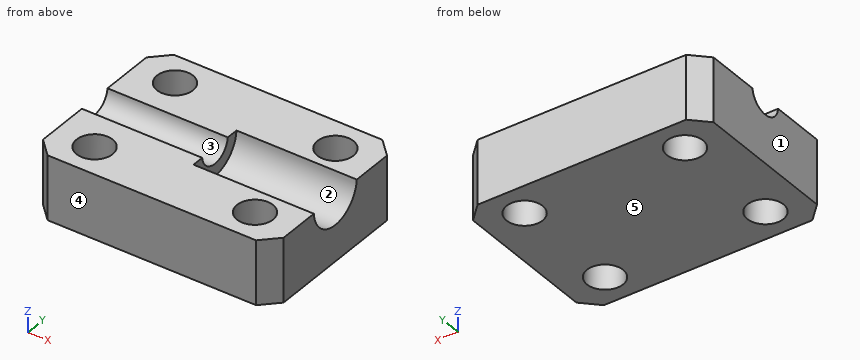
```python
from build123d import *

# Parameters (mm, degrees)
SKETCH2_R           = 2.25
BOSS_EXTRUDE1_DEPTH = 8
CUT_EXTRUDE1_REACH  = 34.939
SKETCH3_R           = 2.25
SKETCH4_R           = 3.75
CUT_EXTRUDE2_DEPTH  = 15


with BuildPart() as part:
    # Sketch2 → Boss-Extrude1 (new body)
    with BuildSketch(Plane.XY):
        Polygon((-13, 11), (13, 11), (15, 9), (15, -9), (13, -11), (-13, -11), (-15, -9), (-15, 9), align=None)
        with Locations((-10, 7)):
            Circle(SKETCH2_R, mode=Mode.SUBTRACT)
        with Locations((-10, -7)):
            Circle(SKETCH2_R, mode=Mode.SUBTRACT)
        with Locations((10, 7)):
            Circle(SKETCH2_R, mode=Mode.SUBTRACT)
        with Locations((10, -7)):
            Circle(SKETCH2_R, mode=Mode.SUBTRACT)
    extrude(amount=BOSS_EXTRUDE1_DEPTH)

    # Sketch3 → Cut-Extrude1 (cut, up to next)
    with BuildSketch(Plane(origin=(15, 0, 0), x_dir=(0, 0, -1), z_dir=(1, 0, 0)), mode=Mode.PRIVATE) as cut_extrude1_sk1:
        with Locations((-8.25, 0)):
            Circle(SKETCH3_R)
    cut_extrude1_tool1 = extrude(cut_extrude1_sk1.sketch, amount=-CUT_EXTRUDE1_REACH, mode=Mode.PRIVATE) & part.part
    add(cut_extrude1_tool1.solids().sort_by_distance((15, 0, 8.25))[0], mode=Mode.SUBTRACT)

    # Sketch4 → Cut-Extrude2 (cut)
    with BuildSketch(Plane(origin=(15, 0, 0), x_dir=(0, 0, -1), z_dir=(1, 0, 0))):
        with Locations((-8.25, 0)):
            Circle(SKETCH4_R)
    extrude(amount=-CUT_EXTRUDE2_DEPTH, mode=Mode.SUBTRACT)


solid = part.part
```
Could you check a few things on this model? Use its own coordinates, in mm. Face numbers are marked on the shaded views. A direction names the side the tool comes from. Round coordinates to 2 decimals unless told otherwise and drop trailing zeros. Loops run counter-clockwise (first coordinate to the right, second up) from the corner with the lowest first, then second, coordinate; pieces in that order, holes last.
Q1. I want a section at D-D (y = 0). Write out the boundary of the cut face in (x, z), and give its area (4 significant figures).
Q2. I want a section at B-B (z = 3.25). Write out the boundary of the cut face in (x, y), and give its area (3 significant figures).
Q3. I want a section at C-C (y = 7). Write out the boundary of the cut face in (x, z), and give its area (3 significant figures).
Q4. On a 3-axis mill with a long thin cutter (end or side, diameter ignored), from which of +Z, -Z, +X, -X, +Y, -Y can I reach the whole of each face in a straight line? I mean the marked faces 1 and 2. Say none if no direction works.
Q5. Thinking about a two-plate mould opening in Y: for the marked faces 3, 4 and 5, which applies, pulls with the +Y half, pulls with the -Y half, needs draft (parallel to the pull), parting line crosses it, or undercut?
Q6. For P1, Ø2.5, axis at x = 10, y = 7, coming from the -Z side; P2, Ø4, axis at y = 1, z = 6, coming from the +X side, each with a flat end and sliding along its axis, tell me the tip position at first contact or that it passes through.
Q7. I want a section at A-A (x = -10). Write out the boundary of the cut face in (y, z).
Q8. Please list where these lines run through material, in increasing order: L1, parallel to Y at x = -10, z = 2.25; L2, parallel to X at y = -5.5, z = 1.5; L3, parallel to Y at x = 11.5, z = 2.
Answer below:
1. outline: (-15, 0) - (15, 0) - (15, 4.5) - (0, 4.5) - (0, 6) - (-15, 6) - close
1. area: 157.5 mm2
2. outline: (-15, -9) - (-13, -11) - (13, -11) - (15, -9) - (15, 9) - (13, 11) - (-13, 11) - (-15, 9) - close; hole circle Ø4.5 at (-10, -7); hole circle Ø4.5 at (-10, 7); hole circle Ø4.5 at (10, -7); hole circle Ø4.5 at (10, 7)
2. area: 588 mm2
3. outline: (-15, 0) - (-12.25, 0) - (-12.25, 8) - (-15, 8) - close; (-7.75, 0) - (7.75, 0) - (7.75, 8) - (-7.75, 8) - close; (12.25, 0) - (15, 0) - (15, 8) - (12.25, 8) - close
3. area: 168 mm2
4. face 1: +Z, -Z, -X, +Y, -Y
4. face 2: +Z, +X
5. face 3: undercut
5. face 4: pulls with the -Y half
5. face 5: needs draft
6. P1: passes through
6. P2: stops at x = 15
7. outline: (-11, 0) - (-9.25, 0) - (-9.25, 8) - (-11, 8) - close; (-4.75, 0) - (4.75, 0) - (4.75, 8) - (2.24, 8) arc R2.25 cw to (-2.24, 8) - (-4.75, 8) - close; (9.25, 0) - (11, 0) - (11, 8) - (9.25, 8) - close
8. L1: y = -11 to -9.25, -4.75 to 4.75, 9.25 to 11
8. L2: x = -15 to -11.68, -8.32 to 8.32, 11.68 to 15
8. L3: y = -11 to -8.68, -5.32 to 5.32, 8.68 to 11
